Geometry: final body of the model. Coordinates: model frame, mm. Face numbers are marked on the shaded views. A direction names the side the tool comes from. Round coordinates to 2 decimals unless told otherwise and drop trailing zeros. Write item = value, one per line. Start each with the question number.
Item 1: Line query: line 1 (Y direction, x = 0.75, z = 0); line 2 (Y direction, x = -3.5, z = 13); line 3 (Y direction, x = 12.5, z = -11). Output: solid intervals per line, ascending. Write a range as from..to.
Item 2: First-contact query: pin 1 (4 mm diameter, centred on y = -1.5, z = -1, fed in from -X); pin 2 (6.5 mm diameter, centred on x = 6.5, y = 16, fed in from -Z); pin 3 (2 mm diameter, centred on x = 10, z = 31.5, fed in from +Y); pin 4 (3 mm diameter, centred on y = 0, z = 0, fed in from -X). Flat tips, straight axial feed; report the tip coordinate or a pass-through.
Item 3: Draft query along Y for the marked faces 3, 4 and 5. Return one class per face: pulls with the +Y half, pulls with the -Y half, needs draft (parallel to the pull), parting line crosses it, or undercut.
Item 4: Access query for the marked faces 1 and 2. Directions: +Z, -Z, +X, -X, +Y, -Y. A direction counts if a zero-diameter tool reaches every point of the face in a straight line with its end or side. Return the directions, or none.
Item 5: Section A-A (z = -15). Count the separate pieces of the cut face and the enclosed holes in it, plus the area to 3 significant figures.
from build123d import *

# Parameters (mm, degrees)
CUT_EXTRUDE1_DEPTH      = 19.5000001
CUT_EXTRUDE1_DEPTH_BACK = 19.5000001


with BuildPart() as part:
    # Sketch1 → Revolve1 (revolve)
    with BuildSketch(Plane(origin=(0, 0, 0), x_dir=(1, 0, 0), z_dir=(0, 1, 0))):
        with BuildLine():
            Line((18.5, -43.576702778), (18.5, -23.576702778))
            Line((18.5, -23.576702778), (4, -7))
            Line((4, -7), (4, -2))
            Line((4, -2), (0, -2))
            Line((0, -2), (0, -46.5))
            ThreePointArc((0, -46.5), (9.364769974, -45.764669773), (18.5, -43.576702778))
        make_face()
    revolve(axis=Axis((-21.521301372, 0, 0), (1, 0, 0)))

    # Mirror1: part across plane


with BuildPart() as part_1:
    add(part.part)
    add(part.part.mirror(Plane(origin=(0, 0, 2), x_dir=(0, 0, 1), z_dir=(-1, 0, 0))))

    # Sketch2 → Cut-Extrude1 (cut, two sides)
    with BuildSketch(Plane(origin=(0, 0, 0), x_dir=(0, 0, -1), z_dir=(1, 0, 0))) as cut_extrude1_sk:
        with BuildLine():
            ThreePointArc((-5.761847074, 3.975062049), (-4.114496766, 5.663118961), (-2, 6.708203932))
            Line((-2, 6.708203932), (-2, 19.474272558))
            ThreePointArc((-2, 19.474272558), (-11.506897181, 15.837885241), (-17.903099827, 7.919994206))
            Line((-17.903099827, 7.919994206), (-5.761847074, 3.975062049))
        make_face()
        with BuildLine():
            Line((2, 19.474272558), (2, 6.708203932))
            ThreePointArc((2, 6.708203932), (4.114496766, 5.663118961), (5.761847074, 3.975062049))
            Line((5.761847074, 3.975062049), (17.903099827, 7.919994206))
            ThreePointArc((17.903099827, 7.919994206), (11.506897181, 15.837885241), (2, 19.474272558))
        make_face()
        with BuildLine():
            Line((-13.064724197, -14.579446948), (-5.56101733, -4.251480479))
            ThreePointArc((-5.56101733, -4.251480479), (-6.657395614, -2.163118961), (-6.997915051, 0.170835984))
            Line((-6.997915051, 0.170835984), (-19.139167805, 4.115768141))
            ThreePointArc((-19.139167805, 4.115768141), (-18.618550745, -6.049533852), (-13.064724197, -14.579446948))
        make_face()
        with BuildLine():
            Line((19.139167805, 4.115768141), (6.997915051, 0.170835984))
            ThreePointArc((6.997915051, 0.170835984), (6.999478743, 0.085424353), (7, 0))
            ThreePointArc((7, 0), (6.630502293, -2.244201271), (5.56101733, -4.251480479))
            Line((5.56101733, -4.251480479), (13.064724197, -14.579446948))
            ThreePointArc((13.064724197, -14.579446948), (17.874723972, -7.983829569), (19.576702778, 0))
            ThreePointArc((19.576702778, 0), (19.467011727, 2.069479659), (19.139167805, 4.115768141))
        make_face()
        with BuildLine():
            Line((9.82865622, -16.930587957), (2.324949352, -6.602621488))
            ThreePointArc((2.324949352, -6.602621488), (0, -7), (-2.324949352, -6.602621488))
            Line((-2.324949352, -6.602621488), (-9.82865622, -16.930587957))
            ThreePointArc((-9.82865622, -16.930587957), (0, -19.576702778), (9.82865622, -16.930587957))
        make_face()
    extrude(amount=CUT_EXTRUDE1_DEPTH, mode=Mode.SUBTRACT)
    extrude(cut_extrude1_sk.sketch, amount=-CUT_EXTRUDE1_DEPTH_BACK, mode=Mode.SUBTRACT)


solid = part_1.part
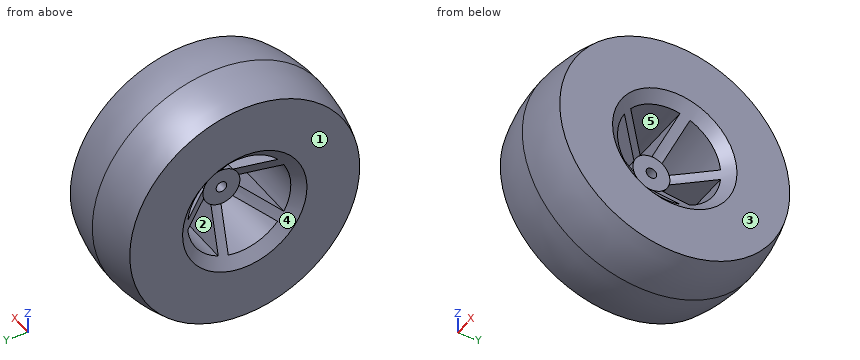
Taken from the geometry:
q1.line_1 = -46.5..-19.58, -7..-2, 2..46.5
q1.line_2 = -44.54..-14.49, 2.12..6.33, 14.64..44.54
q1.line_3 = -43.82..-12.59, 16.19..43.82
q2.pin_1 = -4
q2.pin_2 = -44.41
q2.pin_3 = 34.01
q2.pin_4 = through
q3.face_3 = needs draft
q3.face_4 = undercut
q3.face_5 = undercut
q4.face_1 = +Z, -Z, -X, +Y, -Y
q4.face_2 = +X, -X
q5.separate_pieces = 3
q5.enclosed_holes = 0
q5.area = 2,310 mm^2
